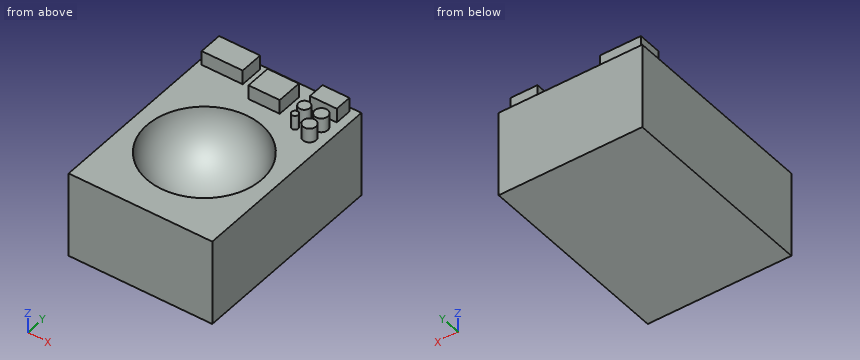
```python
from build123d import *

# Parameters (mm, degrees)
F0_W     = 127
F0_H     = 177.8
F1_DEPTH = 76.2
F4_W     = 36.302225
F4_H     = 20.813279
F4_W_2   = 27.589691
F4_H_2   = 22.749387
F4_W_3   = 23.717456
F4_H_3   = 15.004918
F4_R     = 5.053417
F4_R_2   = 5.808353
F4_R_3   = 2.944236
F4_R_4   = 5.808361
F5_DEPTH = 12.7


with BuildPart() as f1:
    # F0 (on Top) → F1 (new body)
    with BuildSketch(Plane.XY):
        with Locations((0, 12.7)):
            Rectangle(F0_W, F0_H)
    extrude(amount=-F1_DEPTH)

    # F2 (on face) → F3 (revolve, cut)
    with BuildSketch(Plane.XY):
        with BuildLine():
            Line((0, 50.8), (0, -50.8))
            ThreePointArc((0, -50.8), (50.8, 0), (0, 50.8))
        make_face()
    revolve(axis=Axis((0, 0, 0), (0, -1, 0)), mode=Mode.SUBTRACT)

    # F4 (on face) → F5 (join)
    with BuildSketch(Plane.XY):
        with Locations((-41.225782, 87.253075)):
            Rectangle(F4_W, F4_H)
        with Locations((3.788977, 77.572484)):
            Rectangle(F4_W_2, F4_H_2)
        with Locations((43.96344, 90.157256)):
            Rectangle(F4_W_3, F4_H_3)
        with Locations((35.008892, 72.006144)):
            Circle(F4_R)
        with Locations((50.013807, 72.006144)):
            Circle(F4_R_2)
        with Locations((35.008892, 60.87346)):
            Circle(F4_R_3)
        with Locations((50.013807, 57.969283)):
            Circle(F4_R_4)
    extrude(amount=F5_DEPTH)


solid = f1.part
```
Part model, mm, in its own coordinate system. Coordinates: 2 decimals unless noted, no trailing zeros. Order: outer loops, then holes, each group sorted by start corner. A loop starts at its lowest first (then second) coordinate and runs counter-clockwise, first axis right, second up. Notation, with made-up numbers: (48.5, 58) - (104.5, 58) arc R11 ccw to (104.5, 62) - close; hole circle Ø3 at (-11, 20). An arc over 180 degrees is marked (long way). Return JSON: item names as keys, results as strings. Group by question number.
Item 1: Drill centre lines: probe 1 along X at (y, z) = (72, 7); probe 2 along Y at (x, z) = (8.5, -29); probe 3 along Y at (x, z) = (-25.5, 0.5). Where is each one in solid material? Low to high. Write a range as from..to.
Item 2: Cut at A-A (x = -55.5). List the corners of the cut face in (y, z).
Item 3: Cut at B-B (z = -48). List the corners of the cut face in (x, y) (1 decimal).
Item 4: Pin check, flat tips, straight feed: pin 1 (10 mm diameter, centred on y = 92.5, z = 8, fed in from -X); pin 2 (6.5 mm diameter, centred on y = 87, z = 5.5, fed in from +X); pin 3 (10 mm diameter, centred on x = 41.5, z = 3.5, fed in from -Y); pin 4 (10 mm diameter, centred on x = 10, z = 7, fed in from -Y). Stop position of each tip, or through.
Item 5: Cut at C-C (y = -38). List the corners of the cut face in (x, z).
Item 6: Cut at D-D (x = 2.5). List the corners of the cut face in (y, z).
Check values:
{
 "1": {"probe 1": "x = -10.01..17.58, 29.96..40.06, 44.21..55.82", "probe 2": "y = -76.2..-40.83, 40.83..101.6", "probe 3": "y = 76.85..97.66"},
 "2": {"outline": "(-76.2, -76.2) - (101.6, -76.2) - (101.6, 0) - (97.66, 0) - (97.66, 12.7) - (76.85, 12.7) - (76.85, 0) - (-76.2, 0) - close"},
 "3": {"outline": "(-63.5, -76.2) - (63.5, -76.2) - (63.5, 101.6) - (-63.5, 101.6) - close; hole circle Ø33.3 at (0, 0)"},
 "4": {"pin 1": "stops at x = -59.38", "pin 2": "stops at x = 55.82", "pin 3": "stops at y = -76.2", "pin 4": "stops at y = 66.2"},
 "5": {"outline": "(-63.5, -76.2) - (63.5, -76.2) - (63.5, 0) - (33.71, 0) arc R33.71 cw to (-33.71, 0) - (-63.5, 0) - close"},
 "6": {"outline": "(-76.2, -76.2) - (101.6, -76.2) - (101.6, 0) - (88.95, 0) - (88.95, 12.7) - (66.2, 12.7) - (66.2, 0) - (50.74, 0) arc R50.74 cw to (-50.74, 0) - (-76.2, 0) - close"}
}
